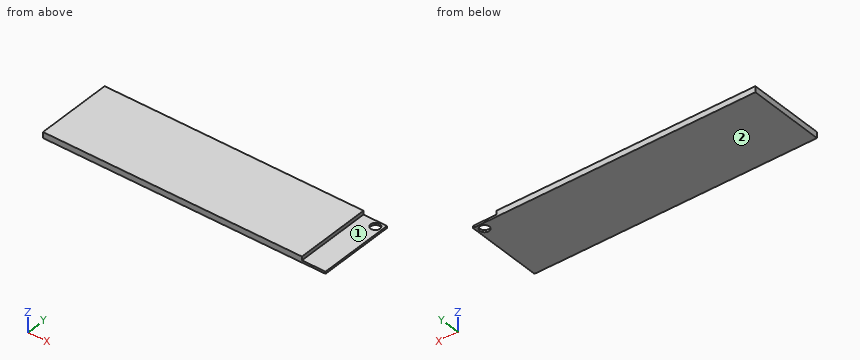
Autodesk Fusion 360 part; units mm, degrees
box "BoxPrimitive1" add length 41.3548 width 139.7 height 3.175 placed x (0, -1, 0) y (1, 0, 0) z (0, 0, 1) at (0, 0, 0)
box "BoxPrimitive2" add length 41.275 width 29.6956 height 1.143 placed x (0, -1, 0) y (1, 0, 0) z (0, 0, 1) at (122.7007, -0.0274, 0)
hole "Hole1" at (148.831, -3.4125, 1.143) direction (0, 0, -1) diameter 5.08 depth 15.24 tip angle 180
CAD build for the part. Positions are in the model's coordinates, mm. Face numbers are marked on the shaded views. A direction names the side the tool comes from. Coordinates: 2 decimals unless noted, no trailing zeros. Write each loop counter-clockwise with the first axis right and the second up, starting at its lowest first coordinate (ties: lowest second). Pieces come first, ordered by that corner, then holes.
(1) Drill centre lines: probe 1 along X at (y, z) = (-32, 2.5); probe 2 along Y at (x, z) = (145, 0.65). Where is each one in solid material? Low to high.
(2) Cut at A-A, the plane y = -30.5. List the corners of the cut face in (x, z) (3 decimals), and give its area (3 significant figures).
(3) Cut at B-B, the plane z = 1.85. List the corners of the cut face in (x, y), and give its area (3 significant figures).
(4) 3-axis set-ups, long thin cutter, end or side, ignore diameter. For the marked faces 1 and 2: which of +Z, -Z, +X, -X, +Y, -Y reach the whole face in a straight line?
(5) Flat gauge pins, fed straight in: pin 1 (0.9 mm diameter, centred on x = 145.5, z = 0.5, fed in from -Y); pin 2 (6.5 mm diameter, centred on x = 148.83, y = -3.41, fed in from +Z); pin 3 (4 mm diameter, centred on x = 55.5, y = -25.5, fed in from -Z). Where does each tip first touch, or does it go through?
Geometry says:
1. probe 1: x = 0 to 139.7
1. probe 2: y = -41.3 to -0.03
2. outline: (0, 0) - (152.396, 0) - (152.396, 1.143) - (139.7, 1.143) - (139.7, 3.175) - (0, 3.175) - close
2. area: 458 mm2
3. outline: (0, -41.35) - (139.7, -41.35) - (139.7, 0) - (0, 0) - close
3. area: 5,780 mm2
4. face 1: +Z, +X, +Y, -Y
4. face 2: -Z, +X, -X, +Y, -Y
5. pin 1: stops at y = -41.3
5. pin 2: stops at z = 1.14
5. pin 3: stops at z = 0
